For this review, use the dimensioned drawing (mm, ordinates from the lowest corner) and the shaded views. A direction names the side the tool comes from. Coordinates: 2 decimals unless noted, no trailing zeros. Order: outer loops, then holes, each group sorted by start corner. A loop starts at its lowest first (then second) coordinate and runs counter-clockwise, first axis right, second up. Notation, with made-up numbers: M 66,-19.75 L 110,-19.75 A13 ccw 110,-7.75 Z; hole C 67.5,87 d10. An arc over 180 degrees is marked long. Answer in a Markdown table with one row per item.
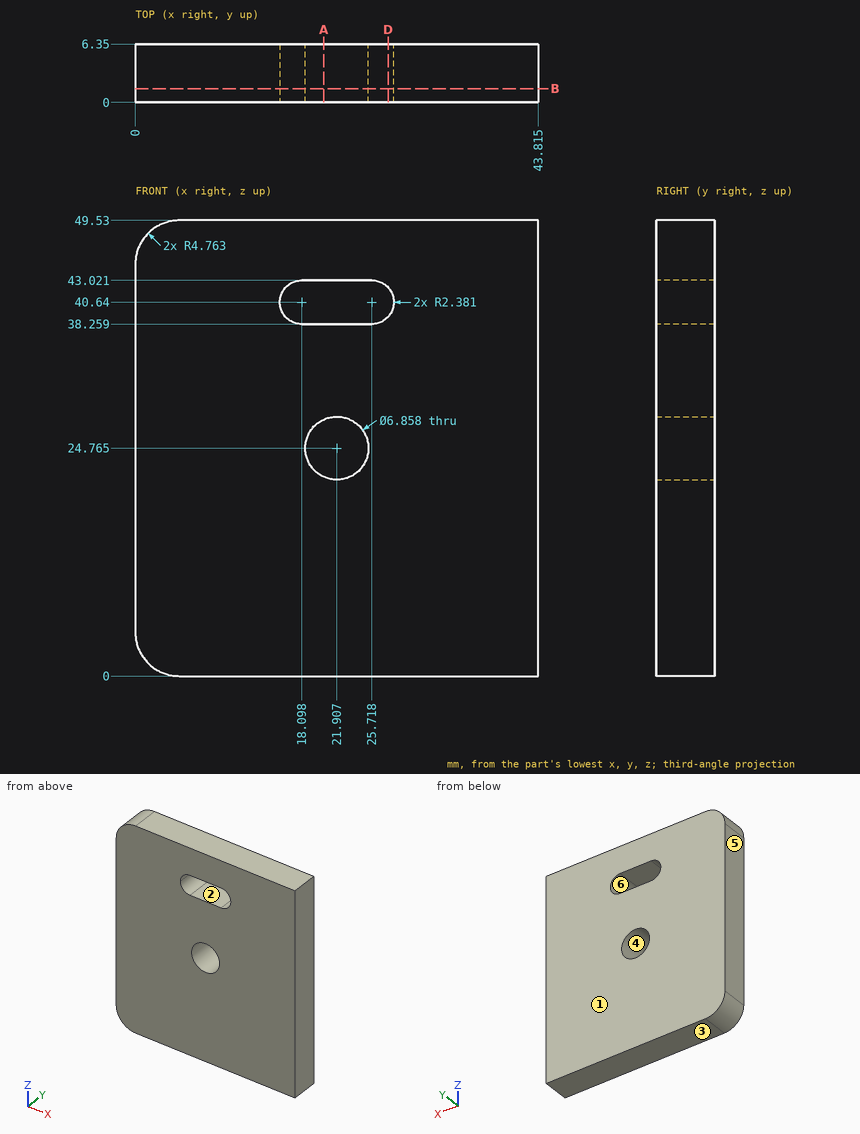
(1) Insertion check: P1, Ø1.5, axis at x = 21, z = 41.5, coming from the +Y side. The pin has a flat end and moves straight along its axis. Give the tip position at first contact, or say it passes through.
Report:
| item | result |
|---|---|
| P1 | through |
(2) The part is to be moulded in two halves that separate along Z. For the marked faces 3, 4, 5 and 6, say which applies: +Z half, -Z half, draft (parallel to the pull), parting line (faces both ways), or undercut.
Report:
| item | result |
|---|---|
| face 3 | -Z half |
| face 4 | undercut |
| face 5 | draft |
| face 6 | undercut |
(3) Take a section at D-D (x = 27.5). Write out the cut boundary in (y, z).
Report:
| item | result |
|---|---|
| outline | M 0,0 L 6.35,0 L 6.35,39.06 L 0,39.06 Z; M 0,42.22 L 6.35,42.22 L 6.35,49.53 L 0,49.53 Z |
(4) Take a section at A-A (x = 20.5). Write out the cut boundary in (y, z).
Report:
| item | result |
|---|---|
| outline | M 0,0 L 6.35,0 L 6.35,21.64 L 0,21.64 Z; M 0,27.89 L 6.35,27.89 L 6.35,38.26 L 0,38.26 Z; M 0,43.02 L 6.35,43.02 L 6.35,49.53 L 0,49.53 Z |
(5) Machinability: for the marked faces 1 and 2, which of the approach directions +Z, -Z, +X, -X, +Y, -Y give a long, thin tool a straight path to every point of the face, cutting with its end or side? Answer none if there is none.
Report:
| item | result |
|---|---|
| face 1 | +Z, -Z, +X, -X, +Y |
| face 2 | +Y, -Y |
(6) Take a section at B-B (y = 1.5). Write out the cut boundary in (x, z) (1 decimal), then the cut area to 3 significant figures.
Report:
| item | result |
|---|---|
| outline | M 0,4.8 A4.8 ccw 4.8,0 L 43.8,0 L 43.8,49.5 L 4.8,49.5 A4.8 ccw 0,44.8 Z; hole M 18.1,38.3 L 25.7,38.3 A2.4 ccw 25.7,43 L 18.1,43 A2.4 ccw Z; hole C 21.9,24.8 d6.9 |
| area | 2,070 mm^2 |
(7) To check wall thickness, follow line 1 (Z direction, x = 20, y = 0.5) (1 decimal); line 2 (Z direction, x = 18, y = 2); line 3 (Z direction, x = 24.5, y = 3.75). State the ranges of each line that lie inside material, in increasing order. Write a range as [from, to].
Report:
| item | result |
|---|---|
| line 1 | [0, 21.9], [27.6, 38.3], [43, 49.5] |
| line 2 | [0, 38.26], [43.02, 49.53] |
| line 3 | [0, 22.52], [27.01, 38.26], [43.02, 49.53] |
